from build123d import *

# Parameters (mm, degrees)
F0_R     = 6
F0_R_2   = 2.5
F1_DEPTH = 5


with BuildPart() as f1:
    # F0 (on Front) → F1 (new body)
    with BuildSketch(Plane.XZ):
        Circle(F0_R)
        Circle(F0_R_2, mode=Mode.SUBTRACT)
    extrude(amount=F1_DEPTH)


with BuildPart() as f2_1:
    # F2: copy of F1
    add(f1.part)


solid = f1.part
For this review, take the finished solid that the model builds, in its own axes (mm). Give positions to 0.01 mm unless a question says otherwise; leave off trailing zeros. Order: outer loops, then holes, each group sorted by start corner. A loop starts at its lowest first (then second) coordinate and runs counter-clockwise, first axis right, second up. Notation, with made-up numbers: (51.5, -7.5) -> (89.5, -7.5) arc R16 ccw to (89.5, 11.5) -> close; hole circle Ø7 at (64, -14.75). An arc over 180 degrees is marked (long way). Write item = value, one per line.
1) We need section D-D, the plane x = -4. Give the boundary of the cut face in (y, z), and give its area (3 significant figures).
Findings:
outline = (-5, -4.47) -> (0, -4.47) -> (0, 4.47) -> (-5, 4.47) -> close
area = 44.7 mm^2
2) We need section C-C, the plane y = -3.4. Give the boundary of the cut face in (x, z).
Findings:
outline = circle Ø12 at (0, 0); hole circle Ø5 at (0, 0)
3) To check wall thickness, follow L1, parallel to Z at x = 0, y = -2.05; L2, parallel to X at y = -2.25, z = 2.25; L3, parallel to Z at x = 0.75, y = -4.3. State the ranges of each line that lie inside material, in increasing order. Write a range as from..to.
Findings:
L1 = -6..-2.5, 2.5..6
L2 = -5.56..-1.09, 1.09..5.56
L3 = -5.95..-2.38, 2.38..5.95
4) We need section B-B, the plane x = 0. Give the boundary of the cut face in (y, z).
Findings:
outline = (-5, -6) -> (0, -6) -> (0, -2.5) -> (-5, -2.5) -> close; (-5, 2.5) -> (0, 2.5) -> (0, 6) -> (-5, 6) -> close
5) Insertion check: pin 1 (3 mm diameter, centred on x = -4.5, y = -2.5, fed in from -Z); pin 2 (1.5 mm diameter, centred on y = -2.5, z = -2.5, fed in from +X); pin 3 (6 mm diameter, centred on x = 2.5, z = -2.5, fed in from +Y). Each pin has a flat end and moves straight along its axis. Give the tip position at first contact, or say it passes through.
Findings:
pin_1 = -5.2
pin_2 = 5.74
pin_3 = 0
6) We need section A-A, the plane z = 0. Give the boundary of the cut face in (x, y), and give its area (3 significant figures).
Findings:
outline = (-6, -5) -> (-2.5, -5) -> (-2.5, 0) -> (-6, 0) -> close; (2.5, -5) -> (6, -5) -> (6, 0) -> (2.5, 0) -> close
area = 35.0 mm^2
